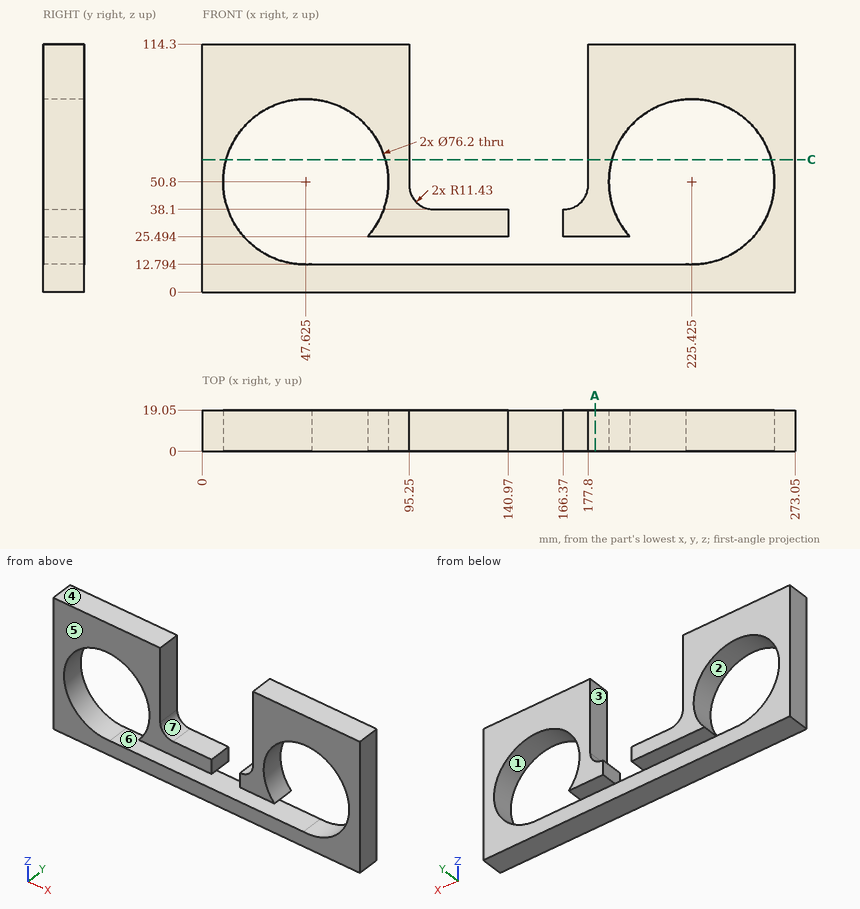
Source: three-view drawing plus pictorial views. Frame: mm from the lowest corner of the part. A direction names the side the tool comes from. Give positions to 0.01 mm unless a question says otherwise; leave off trailing zeros. Loops run counter-clockwise (first coordinate to the right, second up) from the corner with the lowest first, then second, coordinate; pieces in that order, holes last. Notation, with made-up numbers: (35.25, 83.25) -> (60.25, 83.25) arc R24 cw to (60.25, 112.25) -> close; hole circle Ø6 at (-32.5, 53.25). An arc over 180 degrees is marked (long way). Use a Markdown table: item, result. Add a question column.
(1) Section query A-A (x = 181). Output: boundary loops of the cut face in (y, z), then the cut area to 3 significant figures.
(2) Ray query, line 1 (X direction, y = 12.75, z = 50.8) (3 decimals); line 2 (X direction, y = 14, z = 92); line 3 (Z direction, x = 181, y = 3.25). Return the intervals inside material, ascending.
(3) Pull-direction query (Z, two-part tool) for the marked faces 1, 2, 3 and 4; classes: +Z half, -Z half, draft (parallel to the pull), parting line (faces both ways), or undercut.
(4) Access query for the marked faces 5, 6 and 7. Directions: +Z, -Z, +X, -X, +Y, -Y. A direction counts if a zero-diameter tool reaches every point of the face in a straight line with its end or side. Return the directions, or none.
(5) First-contact query: pin 1 Ø5.5 at (x, y) = (140, 13.5) entering from +Z. Flat tip, straight axial feed; report the tip coordinate or a pass-through.
(6) Section query C-C (z = 61). Output: boundary loops of the cut face in (x, y), then the cut area to 3 significant figures.
Checked values:
| question | item | result |
|---|---|---|
| 1 | outline | (0, 0) -> (19.05, 0) -> (19.05, 12.79) -> (0, 12.79) -> close; (0, 25.49) -> (19.05, 25.49) -> (19.05, 114.3) -> (0, 114.3) -> close |
| 1 | area | 1,940 mm^2 |
| 2 | line 1 | 0 to 9.525, 85.725 to 95.25, 177.8 to 187.325, 263.525 to 273.05 |
| 2 | line 2 | 0 to 95.25, 177.8 to 273.05 |
| 2 | line 3 | 0 to 12.79, 25.49 to 114.3 |
| 3 | face 1 | undercut |
| 3 | face 2 | undercut |
| 3 | face 3 | draft |
| 3 | face 4 | +Z half |
| 4 | face 5 | +Z, -Z, +X, -X, -Y |
| 4 | face 6 | +Y, -Y |
| 4 | face 7 | +Z, +Y, -Y |
| 5 | pin 1 | z = 38.1 |
| 6 | outline | (0, 0) -> (10.92, 0) -> (10.92, 19.05) -> (0, 19.05) -> close; (84.33, 0) -> (95.25, 0) -> (95.25, 19.05) -> (84.33, 19.05) -> close; (177.8, 0) -> (188.72, 0) -> (188.72, 19.05) -> (177.8, 19.05) -> close; (262.13, 0) -> (273.05, 0) -> (273.05, 19.05) -> (262.13, 19.05) -> close |
| 6 | area | 832 mm^2 |
